Design review of the part built by this model. Coordinates are the model's own, in mm. Give positions to 0.01 mm unless a question says otherwise; leave off trailing zeros. Loops run counter-clockwise (first coordinate to the right, second up) from the corner with the lowest first, then second, coordinate; pieces in that order, holes last. Notation, with made-up numbers: (41, 5) - (97, 5) arc R18 cw to (97, 34) - close; hole circle Ø6 at (63, -8.75). An arc over 180 degrees is marked (long way). Put each result on its own line as item: value. Start each with the question number.
```python
from build123d import *

# Parameters (mm, degrees)
SKETCH1_W               = 12.7
SKETCH1_H               = 12.7
SKETCH1_W_2             = 9.525
SKETCH1_H_2             = 9.525
BOSS_EXTRUDE1_DEPTH     = 148.59
CUT_EXTRUDE1_DEPTH      = 149.861120176
CUT_EXTRUDE1_DEPTH_BACK = 149.861120176
CUT_EXTRUDE2_DEPTH      = 149.861120176
CUT_EXTRUDE2_DEPTH_BACK = 149.861120176


with BuildPart() as part:
    # Sketch1 → Boss-Extrude1 (new, symmetric)
    with BuildSketch(Plane(origin=(0, 0, 0), x_dir=(0, 0, -1), z_dir=(1, 0, 0))):
        Rectangle(SKETCH1_W, SKETCH1_H)
        Rectangle(SKETCH1_W_2, SKETCH1_H_2, mode=Mode.SUBTRACT)
    extrude(amount=BOSS_EXTRUDE1_DEPTH, both=True)

    # Sketch2 → Cut-Extrude1 (cut, two sides: drawn at the far end of the back side and taken through both)
    with BuildSketch(Plane(origin=(0, 0, 0), x_dir=(1, 0, 0), z_dir=(0, 1, 0)).offset(-CUT_EXTRUDE1_DEPTH_BACK)):
        Polygon((148.59, -6.35), (125.346319759, 26.845415605), (148.59, 26.845415605), align=None)
    extrude(amount=CUT_EXTRUDE1_DEPTH + CUT_EXTRUDE1_DEPTH_BACK, mode=Mode.SUBTRACT)

    # Sketch3 → Cut-Extrude2 (cut, two sides: drawn at the far end of the back side and taken through both)
    with BuildSketch(Plane(origin=(0, 0, 0), x_dir=(1, 0, 0), z_dir=(0, 1, 0)).offset(-CUT_EXTRUDE2_DEPTH_BACK)):
        Polygon((-138.016734859, 6.35), (-148.59, -6.35), (-148.59, 6.35), align=None)
    extrude(amount=CUT_EXTRUDE2_DEPTH + CUT_EXTRUDE2_DEPTH_BACK, mode=Mode.SUBTRACT)


solid = part.part
```
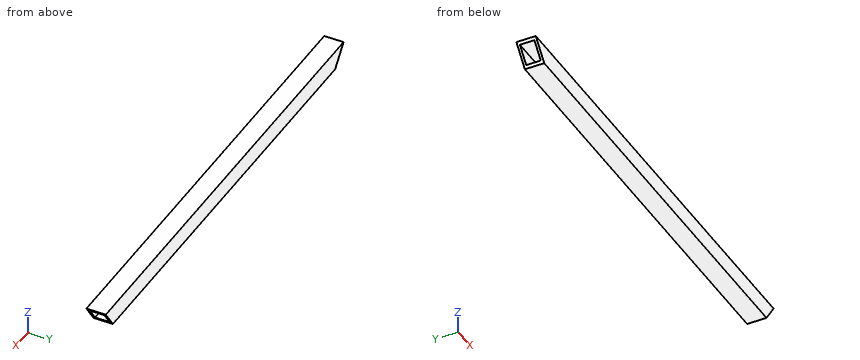
Item 1: Consider section C-C (x = 130.5). State the section outline as (y, z) points, plus the area to 3 significant figures.
Item 2: For L1, parallel to Y at x = -80.5, z = -3.25, list the stretches that pass through material, from the lowest coordinate up. Write a range as from..to.
Item 3: For P1, Ø3, axis at y = -4.5, z = 2, coming from the -X side, flat-tipped, find the tip position at first contact; note if it passes through.
Item 4: Consider section B-B (z = -0.75). State the section outline as (x, y) points.
Item 5: Consider section A-A (y = 0). State the section outline as (x, z) points, plus the area to 3 significant figures.
Geometry says:
1. outline: (-6.35, -6.35) - (6.35, -6.35) - (6.35, 6.35) - (-6.35, 6.35) - close; hole (-4.76, -4.76) - (4.76, -4.76) - (4.76, 4.76) - (-4.76, 4.76) - close
1. area: 70.6 mm2
2. L1: y = -6.35..-4.76, 4.76..6.35
3. P1: stops at x = -146.2
4. outline: (-142.68, -6.35) - (143.62, -6.35) - (143.62, -4.76) - (-142.68, -4.76) - close; (-142.68, 4.76) - (143.62, 4.76) - (143.62, 6.35) - (-142.68, 6.35) - close
5. outline: (-148.59, 6.35) - (-147.27, 4.76) - (147.48, 4.76) - (148.59, 6.35) - close; (-139.34, -4.76) - (-138.02, -6.35) - (139.7, -6.35) - (140.81, -4.76) - close
5. area: 913 mm2
